Verification items for the finished model (mm, model axes). A direction names the side the tool comes from. Round coordinates to 2 decimals unless told otherwise and drop trailing zeros. Order: outer loops, then holes, each group sorted by start corner. A loop starts at its lowest first (then second) coordinate and runs counter-clockwise, first axis right, second up. Notation, with made-up numbers: (38, 43) -> (60, 43) arc R22 ccw to (60, 72) -> close; hole circle Ø6 at (22, -5). An arc over 180 degrees is marked (long way). Answer in a Markdown table with one row per item. Add a question column.
```python
from build123d import *

# Parameters (mm, degrees)
BOSS_EXTRUDE1_DEPTH = 25.4
FILLET4_R           = 2.54
FILLET5_R           = 2.54


with BuildPart() as part:
    # Sketch2 → Boss-Extrude1 (new body)
    with BuildSketch(Plane.XY):
        with BuildLine():
            Line((0, 0), (0, 92.075))
            Line((0, 92.075), (18.075, 92.075))
            Line((18.075, 92.075), (18.075, 81.825))
            ThreePointArc((18.075, 81.825), (28.325, 71.575), (38.575, 81.825))
            Line((38.575, 81.825), (38.575, 92.075))
            Line((38.575, 92.075), (57.15, 92.075))
            Line((57.15, 92.075), (57.15, 76.835))
            Line((57.15, 76.835), (88.9, 76.835))
            Line((88.9, 76.835), (88.9, 0))
            Line((88.9, 0), (0, 0))
        make_face()
    extrude(amount=BOSS_EXTRUDE1_DEPTH)

    # Fillet4
    fillet4_edges = [part.edges().sort_by_distance(p)[0] for p in [
        (0, 46.0375, 0),
        (9.0375, 92.075, 0),
        (18.075, 86.95, 0),
        (28.325, 71.575, 0),
        (38.575, 86.95, 0),
        (47.8625, 92.075, 0),
        (57.15, 84.455, 0),
        (73.025, 76.835, 25.4),
        (73.025, 76.835, 0),
        (88.9, 38.4175, 0),
        (57.15, 84.455, 25.4),
        (88.9, 76.835, 12.7),
        (47.8625, 92.075, 25.4),
        (38.575, 86.95, 25.4),
        (28.325, 71.575, 25.4),
        (18.075, 86.95, 25.4),
        (9.0375, 92.075, 25.4),
        (0, 46.0375, 25.4),
        (88.9, 38.4175, 25.4),
    ]]
    fillet(fillet4_edges, radius=FILLET4_R)

    # Fillet5
    # the kernel refuses this fillet: 2.54 mm, written as the material it takes off along each edge
    with BuildSketch(Plane(origin=(2.54, 89.535, 22.86), x_dir=(0, 1, 0), z_dir=(-1, 0, 0))) as fillet5_piece_1_section:
        Polygon((0, 0), (FILLET5_R, 0), (FILLET5_R, -FILLET5_R), (0, -FILLET5_R), align=None)
    fillet5_piece_1 = extrude(amount=FILLET5_R, mode=Mode.PRIVATE)
    fillet5_piece_1 = fillet5_piece_1 - Plane(origin=(2.54, 89.535, 22.86), x_dir=(0, -0.7071067811865475, -0.7071067811865475), z_dir=(-1, 0, 0)) * Sphere(FILLET5_R, mode=Mode.PRIVATE)
    add(fillet5_piece_1, mode=Mode.SUBTRACT)
    with BuildSketch(Plane(origin=(54.61, 89.535, 22.86), x_dir=(0, 1, 0), z_dir=(1, 0, 0))) as fillet5_piece_2_section:
        Polygon((0, 0), (FILLET5_R, 0), (FILLET5_R, FILLET5_R), (0, FILLET5_R), align=None)
    fillet5_piece_2 = extrude(amount=FILLET5_R, mode=Mode.PRIVATE)
    fillet5_piece_2 = fillet5_piece_2 - Plane(origin=(54.61, 89.535, 22.86), x_dir=(0, -0.7071067811865475, -0.7071067811865475), z_dir=(1, 0, 0)) * Sphere(FILLET5_R, mode=Mode.PRIVATE)
    add(fillet5_piece_2, mode=Mode.SUBTRACT)
    with BuildSketch(Plane(origin=(2.54, 89.535, 2.54), x_dir=(0, 1, 0), z_dir=(-1, 0, 0))) as fillet5_piece_3_section:
        Polygon((0, 0), (FILLET5_R, 0), (FILLET5_R, FILLET5_R), (0, FILLET5_R), align=None)
    fillet5_piece_3 = extrude(amount=FILLET5_R, mode=Mode.PRIVATE)
    fillet5_piece_3 = fillet5_piece_3 - Plane(origin=(2.54, 89.535, 2.54), x_dir=(0, -0.7071067811865475, 0.7071067811865475), z_dir=(-1, 0, 0)) * Sphere(FILLET5_R, mode=Mode.PRIVATE)
    add(fillet5_piece_3, mode=Mode.SUBTRACT)
    with BuildSketch(Plane(origin=(54.61, 89.535, 2.54), x_dir=(0, 1, 0), z_dir=(1, 0, 0))) as fillet5_piece_4_section:
        Polygon((0, 0), (FILLET5_R, 0), (FILLET5_R, -FILLET5_R), (0, -FILLET5_R), align=None)
    fillet5_piece_4 = extrude(amount=FILLET5_R, mode=Mode.PRIVATE)
    fillet5_piece_4 = fillet5_piece_4 - Plane(origin=(54.61, 89.535, 2.54), x_dir=(0, -0.7071067811865475, 0.7071067811865475), z_dir=(1, 0, 0)) * Sphere(FILLET5_R, mode=Mode.PRIVATE)
    add(fillet5_piece_4, mode=Mode.SUBTRACT)
    with BuildSketch(Plane(origin=(0, 92.075, 2.54), x_dir=(0, -1, 0), z_dir=(0, 0, 1))) as fillet5_piece_5:
        with BuildLine():
            CenterArc((FILLET5_R, FILLET5_R), FILLET5_R, 180, 90)
            Line((0, FILLET5_R), (0, 0))
            Line((0, 0), (FILLET5_R, 0))
        make_face()
    extrude(amount=20.32, mode=Mode.SUBTRACT)
    with BuildSketch(Plane(origin=(57.15, 92.075, 2.54), x_dir=(0, -1, 0), z_dir=(0, 0, 1))) as fillet5_piece_6:
        with BuildLine():
            CenterArc((FILLET5_R, -FILLET5_R), FILLET5_R, 90, 90)
            Line((0, -FILLET5_R), (0, 0))
            Line((0, 0), (FILLET5_R, 0))
        make_face()
    extrude(amount=20.32, mode=Mode.SUBTRACT)


solid = part.part
```
1) Cross-section at A-A, the plane z = 18.25. Record the boundary of the cut face in (x, y) (3 decimals), and give its area (3 significant figures).
2) Cross-section at B-B, the plane x = 60. Record the boundary of the cut face in (y, z) (3 decimals).
3) Tool access check on faces 1 (the face through (72, 76.835, 13)), 2 (the face through (39.299, 87.022, 0.764)), 3 (the face through (56.426, 81.808, 0.764)). Record the directions out of +Z, -Z, +X, -X, +Y, -Y that give a thin tool (end or side, any length) a straight path to the whole face; none if there is none.
4) Draft check along X on faces 4 (the face through (10.416, 91.351, 0.764)), 5 (the face through (28.1, 71.577, 12.558)), 6 (the face through (56.426, 81.808, 24.636)), 7 (the face through (18.075, 87, 13)). Enter one of: +X half, -X half, draft (parallel to the pull), parting line (faces both ways), or undercut.
5) Thickness scan on L1, parallel to Y at x = 73.5, z = 21.25 (3 decimals); L2, parallel to X at y = 77, z = 15.25; L3, parallel to Y at x = 28, z = 6.25. Record the ranges inside material, lowest first. Write a range as [from, to].
6) Depth check by flat-ended pin: P1, Ø8, axis at x = 71, z = 22.5, coming from the -Y side; P2, Ø11.5, axis at y = 86.5, z = 15, coming from the +X side; P3, Ø6, axis at x = 64.5, z = 14.5, coming from the +Y side (3 decimals). Enter the tip coordinate at first touch or a pass-through.
Results below:
| question | item | result |
|---|---|---|
| 1 | outline | (0, 0) -> (88.9, 0) -> (88.9, 74.295) arc R2.54 ccw to (86.36, 76.835) -> (57.15, 76.835) -> (57.15, 89.535) arc R2.54 ccw to (54.61, 92.075) -> (38.575, 92.075) -> (38.575, 81.825) arc R10.25 cw to (18.075, 81.825) -> (18.075, 92.075) -> (2.54, 92.075) arc R2.54 ccw to (0, 89.535) -> close |
| 1 | area | 7,320 mm² |
| 2 | outline | (0, 0) -> (74.295, 0) arc R2.54 ccw to (76.835, 2.54) -> (76.835, 22.86) arc R2.54 ccw to (74.295, 25.4) -> (0, 25.4) -> close |
| 3 | face 1 | +Z, -Z, +X, +Y |
| 3 | face 2 | -Z, +Y |
| 3 | face 3 | -Z, +X, +Y |
| 4 | face 4 | draft |
| 4 | face 5 | undercut |
| 4 | face 6 | +X half |
| 4 | face 7 | undercut |
| 5 | L1 | [0, 76.835] |
| 5 | L2 | [0, 19.28], [37.37, 57.15] |
| 5 | L3 | [0, 71.58] |
| 6 | P1 | y = 0 |
| 6 | P2 | x = 57.15 |
| 6 | P3 | y = 76.835 |
